from build123d import *

# Parameters (mm, degrees)
BOSS_EXTRUDE1_DEPTH = 2.875


with BuildPart() as part:
    # Sketch1 → Boss-Extrude1 (new body, symmetric)
    with BuildSketch(Plane.XY):
        with BuildLine():
            Line((-11.98, -13.98), (11.98, -13.98))
            Line((11.98, -13.98), (11.98, 0))
            ThreePointArc((11.98, 0), (10.378283744, 5.984281622), (6.001431298, 10.368376072))
            ThreePointArc((6.001431298, 10.368376072), (3.951789306, 9.821596677), (4.498568702, 7.771954685))
            ThreePointArc((4.498568702, 7.771954685), (4.485713603, -7.779381304), (-8.98, 0))
            ThreePointArc((-8.98, 0), (-7.779381304, 4.485713603), (-4.498568702, 7.771954685))
            ThreePointArc((-4.498568702, 7.771954685), (-3.951789306, 9.821596677), (-6.001431298, 10.368376072))
            ThreePointArc((-6.001431298, 10.368376072), (-10.378283744, 5.984281622), (-11.98, 0))
            Line((-11.98, 0), (-11.98, -13.98))
        make_face()
    extrude(amount=BOSS_EXTRUDE1_DEPTH, both=True)

    # Sketch4 one side → Cut-Revolve1 (revolve, cut)
    with BuildSketch(Plane.XY):
        Polygon((-1.5, -13.98), (0, -13.98), (0, -7.48), (-2.9, -7.48), (-2.9, -12.48), (-1.5, -12.48), align=None)
    revolve(axis=Axis((0, -13.98, 0), (0, 1, 0)), mode=Mode.SUBTRACT)


solid = part.part
The listing builds one solid part. Answer for the finished solid, in the listing's coordinates (mm). A direction names the side the tool comes from. Round coordinates to 2 decimals unless told otherwise and drop trailing zeros. Write each loop counter-clockwise with the first axis right and the second up, starting at its lowest first coordinate (ties: lowest second). Pieces come first, ordered by that corner, then holes. Notation, with made-up numbers: M 64.25,1.5 L 92.25,1.5 A20 ccw 92.25,36.5 Z; hole C 43.5,79 d6. An arc over 180 degrees is marked long. Write each question's results on one line, items separated by ' | '. Start each with the question number.
(1) The part is cut by section B-B, the plane z = 0. Write down the section's boundary in (x, y), and give its area (3 significant figures).
(2) Find the intervals of material crossed by line 1 (Z direction, x = 0, y = -13.35) (3 decimals); line 2 (X direction, y = 7, z = 2.6); line 3 (Y direction, x = 4.5, z = -0.95), in increasing order.
(3) Determine the mould class of faces 1 (the cylindrical face through (2.9, -10.5, 0.1)), 2 (the cylindrical face through (10.42, 5.91, 0.04)), 3 (the flat face through (-11.98, -7, 0)), 4 (the flat face through (-3, -10, 2.875)) for opening direction X: +X half, -X half, draft (parallel to the pull), parting line (faces both ways), or undercut.
(4) Each of these flat-tipped pins is pushed along its axis until it touches: P1, Ø2, axis at x = -5.5, y = 3.5, coming from the -Z side; P2, Ø3, axis at y = 5.5, z = 0, coming from the -X side. Where does it stop, or does it pass through?
(5) The part is cut by section C-C, the plane y = 3. Write down the section's boundary in (x, z) (3 decimals).
(6) The part is cut by section A-A, the plane x = 0. Write down the section's boundary in (y, z) (3 decimals).
(7) The part is cut by section D-D, the plane z = 2.2. Write down the section's boundary in (x, y), and give its area (3 significant figures).
(8) For faces 5 (the flat face through (0, -13.98, -2)), 6 (the cylindrical face through (8.757, -1.987, -0.04)), 7 (the flat face through (-1.2, -12.48, -1.2)), determine the directions among +Z, -Z, +X, -X, +Y, -Y from which every point of the face is accessible in a straight line to the end or side of a thin tool.
Worked answers:
1) outline: M -11.98,-13.98 L -1.5,-13.98 L -1.5,-12.48 L -2.9,-12.48 L -2.9,-8.5 A8.98 cw -4.5,7.77 A1.5 ccw -6,10.37 A11.98 ccw -11.98,0 Z; M 1.5,-13.98 L 11.98,-13.98 L 11.98,0 A11.98 ccw 6,10.37 A1.5 ccw 4.5,7.77 A8.98 cw 2.9,-8.5 L 2.9,-12.48 L 1.5,-12.48 Z | area: 255 mm²
2) line 1: z = -2.875 to -1.5, 1.5 to 2.875 | line 2: x = -9.72 to -5.62, 5.62 to 9.72 | line 3: y = -13.98 to -7.77, 7.77 to 10.37
3) face 1: undercut | face 2: +X half | face 3: -X half | face 4: draft
4) P1: passes through | P2: stops at x = -11.29
5) outline: M -11.598,-2.875 L -8.464,-2.875 L -8.464,2.875 L -11.598,2.875 Z; M 8.464,-2.875 L 11.598,-2.875 L 11.598,2.875 L 8.464,2.875 Z
6) outline: M -13.98,-2.875 L -12.48,-2.875 L -12.48,-1.5 L -13.98,-1.5 Z; M -13.98,1.5 L -12.48,1.5 L -12.48,2.875 L -13.98,2.875 Z
7) outline: M -11.98,-13.98 L 11.98,-13.98 L 11.98,0 A11.98 ccw 6,10.37 A1.5 ccw 4.5,7.77 A8.98 cw 1.89,-8.78 L 1.89,-12.48 L -1.89,-12.48 L -1.89,-8.78 A8.98 cw -4.5,7.77 A1.5 ccw -6,10.37 A11.98 ccw -11.98,0 Z | area: 268 mm²
8) face 5: +Z, -Z, +X, -X, -Y | face 6: +Z, -Z | face 7: +Y
